Source: CAD feature listing. Evaluate the final solid. Frame: model axes, mm. A direction names the side the tool comes from. Give positions to 0.01 mm unless a question says otherwise; leave off trailing zeros. Loops run counter-clockwise (first coordinate to the right, second up) from the corner with the lowest first, then second, coordinate; pieces in that order, holes last. Notation, with made-up numbers: (82.5, 71) - (119.5, 71) arc R19 cw to (119.5, 102) - close; hole circle Ø6 at (48, 41.25). An arc over 180 degrees is marked (long way). Put each result on its own line as item: value.
```python
from build123d import *

# Parameters (mm, degrees)
EXTRUDE_1_DEPTH     = 5
SKETCH_2_W          = 6.5
SKETCH_2_H          = 14
CUT_EXTRUDE_1_DEPTH = 5
SKETCH_3_R          = 1.4
CUT_EXTRUDE_2_DEPTH = 45.877611345
FILLET_1_R          = 5
CUT_EXTRUDE_START   = -1
CUT_EXTRUDE_5_DEPTH = 1


with BuildPart() as part:
    # 草图1 → 凸台-拉伸1 (new body)
    with BuildSketch(Plane.XY):
        Polygon((30, 0), (-30, 0), (-30, 11.5), (-21, 11.5), (-21, 33), (21, 33), (21, 11.5), (30, 11.5), align=None)
    extrude(amount=EXTRUDE_1_DEPTH)

    # 草图2 → 切除-拉伸1 (cut)
    with BuildSketch(Plane(origin=(0, 0, 0), x_dir=(-1, 0, 0), z_dir=(0, 0, -1))):
        with Locations((-9.75, 15.5)):
            Rectangle(SKETCH_2_W, SKETCH_2_H)
        with Locations((9.75, 15.5)):
            Rectangle(SKETCH_2_W, SKETCH_2_H)
    extrude(amount=-CUT_EXTRUDE_1_DEPTH, mode=Mode.SUBTRACT)

    # 草图3 → 切除-拉伸2 (cut, through all)
    with BuildSketch(Plane(origin=(0, 0, 0), x_dir=(-1, 0, 0), z_dir=(0, 0, -1))):
        with Locations((-25.1, 3)):
            Circle(SKETCH_3_R)
        with Locations((-15.2, 26.6)):
            Circle(SKETCH_3_R)
        with Locations((25.1, 3)):
            Circle(SKETCH_3_R)
        with Locations((15.2, 26.6)):
            Circle(SKETCH_3_R)
    extrude(amount=-CUT_EXTRUDE_2_DEPTH, mode=Mode.SUBTRACT)

    # 圆角1
    fillet_1_edges = [part.edges().sort_by_distance(p)[0] for p in [
        (-21, 11.5, 2.5),
        (21, 11.5, 2.5),
    ]]
    fillet(fillet_1_edges, radius=FILLET_1_R)

    # 草图5 → 切除-拉伸5 (cut)
    with BuildSketch(Plane(origin=(0, 0, 0), x_dir=(-1, 0, 0), z_dir=(0, 0, -1)).offset(CUT_EXTRUDE_START)):
        with BuildLine():
            Line((21, 33), (-21, 33))
            Line((-21, 33), (-21, 16.5))
            ThreePointArc((-21, 16.5), (-22.464466094, 12.964466094), (-26, 11.5))
            Line((-26, 11.5), (-30, 11.5))
            Line((-30, 11.5), (-30, 0))
            Line((-30, 0), (-28, 0))
            Line((-28, 0), (-28, 10.5))
            Line((-28, 10.5), (-19, 10.5))
            Line((-19, 10.5), (-19, 31))
            Line((-19, 31), (19, 31))
            Line((19, 31), (19, 10.5))
            Line((19, 10.5), (28, 10.5))
            Line((28, 10.5), (28, 0))
            Line((28, 0), (30, 0))
            Line((30, 0), (30, 11.5))
            Line((30, 11.5), (26, 11.5))
            ThreePointArc((26, 11.5), (22.464466094, 12.964466094), (21, 16.5))
            Line((21, 16.5), (21, 33))
        make_face()
    extrude(amount=CUT_EXTRUDE_5_DEPTH, mode=Mode.SUBTRACT)


solid = part.part
```
1) Material intervals for line 1 along X through (y, z) = (16.5, 0.25); line 2 along X through (y, z) = (18.5, 4.1); line 3 along Y through (x, z) = (-15.2, 3.2), sorted ascending. Write a range as [from, to].
Check result:
line 1: [-19, -13], [-6.5, 6.5], [13, 19]
line 2: [-21, -13], [-6.5, 6.5], [13, 21]
line 3: [0, 25.2], [28, 33]
2) Pin query (flat end, axial travel): P1, Ø0.5, axis at y = 5.5, z = 0.5, coming from the +X side; P2, Ø0.8, axis at y = 24.5, z = 0.5, coming from the +X side; P3, Ø1, axis at y = 19.5, z = 2, coming from the +X side; P4, Ø2.5, axis at x = -15.2, y = 26.6, coming from the -Z side. Return the tip coordinate at first contact, or that it passes through.
Check result:
P1: x = 28
P2: x = 19
P3: x = 21
P4: through
3) Section query A-A, the plane y = 13.5. Output: boundary loops of the cut face in (x, z), plus the area to 3 significant figures.
Check result:
outline: (-22, 1) - (-19, 1) - (-19, 0) - (-13, 0) - (-13, 5) - (-22, 5) - close; (-6.5, 0) - (6.5, 0) - (6.5, 5) - (-6.5, 5) - close; (13, 0) - (19, 0) - (19, 1) - (22, 1) - (22, 5) - (13, 5) - close
area: 149 mm²
4) Section query C-C, the plane x = 15.2. Output: boundary loops of the cut face in (y, z), plus the area to 3 significant figures.
Check result:
outline: (0, 0) - (25.2, 0) - (25.2, 5) - (0, 5) - close; (28, 0) - (31, 0) - (31, 1) - (33, 1) - (33, 5) - (28, 5) - close
area: 149 mm²
5) Section query D-D, the plane y = 30. Output: boundary loops of the cut face in (x, z).
Check result:
outline: (-21, 1) - (-19, 1) - (-19, 0) - (19, 0) - (19, 1) - (21, 1) - (21, 5) - (-21, 5) - close
6) Access query for faces 1 (the flat face through (0, 0, 2)), 2 (the flat face through (-6.5, 15, 2)), 3 (the flat face through (28, 11.5, 3)). Directions: +Z, -Z, +X, -X, +Y, -Y. A direction counts if a zero-diameter tool reaches every point of the face in a straight line with its end or side. Return the directions, or none.
Check result:
face 1: +Z, -Z, +X, -X, -Y
face 2: +Z, -Z
face 3: +Z, -Z, +X, +Y
7) Mould query, pull axis X, two halves, no side actions, for faces 4 (the flat face through (21, 25, 3)), 5 (the flat face through (-28, 11.5, 3)), 6 (the cylindrical face through (23.81, 2.46, 2.46)). Classes: pulls with the +X half, pulls with the -X half, needs draft (parallel to the pull), parting line crosses it, or undercut.
Check result:
face 4: pulls with the +X half
face 5: needs draft
face 6: undercut
8) Section query B-B, the plane z = 3.2. Output: boundary loops of the cut face in (x, y).
Check result:
outline: (-30, 0) - (30, 0) - (30, 11.5) - (26, 11.5) arc R5 cw to (21, 16.5) - (21, 33) - (-21, 33) - (-21, 16.5) arc R5 cw to (-26, 11.5) - (-30, 11.5) - close; hole circle Ø2.8 at (-25.1, 3); hole circle Ø2.8 at (-15.2, 26.6); hole (-13, 8.5) - (-6.5, 8.5) - (-6.5, 22.5) - (-13, 22.5) - close; hole (6.5, 8.5) - (13, 8.5) - (13, 22.5) - (6.5, 22.5) - close; hole circle Ø2.8 at (15.2, 26.6); hole circle Ø2.8 at (25.1, 3)
